Source: CAD feature listing. Evaluate the final solid. Frame: model axes, mm. A direction names the side the tool comes from. Give positions to 0.01 mm unless a question says otherwise; leave off trailing zeros. Loops run counter-clockwise (first coordinate to the right, second up) from the corner with the lowest first, then second, coordinate; pieces in that order, holes last. Notation, with made-up numbers: (-16.5, 16) - (-7.5, 16) arc R33 cw to (-7.5, 48) - close; hole circle Ø7 at (44.25, 74.25). An arc over 180 degrees is marked (long way). Put each result on its own line as item: value.
```python
from build123d import *

# Parameters (mm, degrees)
BASE_FLANGE1_DEPTH              = 3
EDGE_FLANGE1_STRIP_W            = 13.4732
EDGE_FLANGE1_STRIP_H            = 3
EDGE_FLANGE1_STRIP_CUT_DEPTH    = 80
EDGE_FLANGE1_RELIEF_W           = 14.9732
EDGE_FLANGE1_RELIEF_H           = 1.5
EDGE_FLANGE1_RELIEF_CUT_DEPTH   = 3
EDGE_FLANGE1_STRIP_2_W          = 13.4732
EDGE_FLANGE1_STRIP_2_H          = 3
EDGE_FLANGE1_STRIP_CUT_2_DEPTH  = 80
EDGE_FLANGE1_RELIEF_2_W         = 14.9732
EDGE_FLANGE1_RELIEF_2_H         = 1.5
EDGE_FLANGE1_RELIEF_CUT_2_DEPTH = 3
EDGE_FLANGE1_DEPTH              = 80
EDGE_FLANGE1_BEND_DEPTH         = 80
HEM1_START                      = -51.311042424
HEM1_DEPTH                      = 80
HEM1_2_DEPTH                    = 80
EDGE_FLANGE2_STRIP_W            = 13.4732
EDGE_FLANGE2_STRIP_H            = 3
EDGE_FLANGE2_STRIP_CUT_DEPTH    = 80
EDGE_FLANGE2_STRIP_2_W          = 13.4732
EDGE_FLANGE2_STRIP_2_H          = 3
EDGE_FLANGE2_STRIP_CUT_2_DEPTH  = 80
EDGE_FLANGE2_DEPTH              = 80
EDGE_FLANGE2_BEND_DEPTH         = 80
CHAMFER1_SIZE                   = 10
SKETCH24_W                      = 40
SKETCH24_H                      = 20
CUT_EXTRUDE1_DEPTH              = 3
SKETCH25_R                      = 2.58
CUT_EXTRUDE3_DEPTH              = 3
CUT_EXTRUDE2_START              = -3
CUT_EXTRUDE2_OUTLINE_W          = 79.5268
CUT_EXTRUDE2_OUTLINE_H          = 20
CUT_EXTRUDE2_DEPTH              = 3


# Read off the part's stored shape, not the designer's step: Hem1, Cut-Extrude2
# Sheet-metal steps are written as plain solids
with BuildPart() as part:
    # Sketch1 → Base-Flange1 (new body)
    with BuildSketch(Plane(origin=(0, 0, 0), x_dir=(1, 0, 0), z_dir=(0, 1, 0))):
        Polygon((-40.5, 51.311042424), (-40.5, -28.688957576), (40.5, -28.688957576), (40.5, 51.311042424), (40, 51.311042424), (40, 73.311042424), (-40, 73.311042424), (-40, 51.311042424), align=None)
    extrude(amount=-BASE_FLANGE1_DEPTH)

    # Edge-Flange1 strip (across the edge) → Edge-Flange1 strip cut (cut)
    with BuildSketch(Plane(origin=(40.5, 0, 28.688957576), x_dir=(-1, 0, 0), z_dir=(0, 0, -1))):
        with Locations((-6, -1.5)):
            Rectangle(EDGE_FLANGE1_STRIP_W, EDGE_FLANGE1_STRIP_H)
    extrude(amount=EDGE_FLANGE1_STRIP_CUT_DEPTH, mode=Mode.SUBTRACT)

    # Edge-Flange1 relief (on the sheet) → Edge-Flange1 relief cut (cut)
    with BuildSketch(Plane(origin=(39.7634, 0, 28.688957576), x_dir=(-1, 0, 0), z_dir=(0, 1, 0))):
        with Locations((-5.9866, -80.75)):
            Rectangle(EDGE_FLANGE1_RELIEF_W, EDGE_FLANGE1_RELIEF_H)
    extrude(amount=-EDGE_FLANGE1_RELIEF_CUT_DEPTH, mode=Mode.SUBTRACT)

    # Edge-Flange1 strip 2 (across the edge) → Edge-Flange1 strip cut 2 (cut)
    with BuildSketch(Plane(origin=(-40.5, 0, -51.311042424), x_dir=(1, 0, 0), z_dir=(0, 0, 1))):
        with Locations((-6, -1.5)):
            Rectangle(EDGE_FLANGE1_STRIP_2_W, EDGE_FLANGE1_STRIP_2_H)
    extrude(amount=EDGE_FLANGE1_STRIP_CUT_2_DEPTH, mode=Mode.SUBTRACT)

    # Edge-Flange1 relief 2 (on the sheet) → Edge-Flange1 relief cut 2 (cut)
    with BuildSketch(Plane(origin=(-39.7634, 0, -51.311042424), x_dir=(1, 0, 0), z_dir=(0, 1, 0))):
        with Locations((-5.9866, 0.75)):
            Rectangle(EDGE_FLANGE1_RELIEF_2_W, EDGE_FLANGE1_RELIEF_2_H)
    extrude(amount=-EDGE_FLANGE1_RELIEF_CUT_2_DEPTH, mode=Mode.SUBTRACT)

    # Edge-Flange1 section (across the edge) → Edge-Flange1 (add)
    with BuildSketch(Plane(origin=(40.5, 0, 28.688957576), x_dir=(-1, 0, 0), z_dir=(0, 0, -1))):
        with BuildLine():
            Line((-3, 0.7366), (-3, 5))
            Line((-3, 5), (0, 5))
            Line((0, 5), (0, 0.7366))
            ThreePointArc((0, 0.7366), (0.215745145, 0.215745145), (0.7366, 0))
            Line((0.7366, 0), (0.7366, -3))
            ThreePointArc((0.7366, -3), (-1.905575199, -1.905575199), (-3, 0.7366))
        make_face()
    extrude(amount=EDGE_FLANGE1_DEPTH)

    # Edge-Flange1 section 2 (across the edge) → Edge-Flange1 bend (add)
    with BuildSketch(Plane(origin=(-40.5, 0, -51.311042424), x_dir=(1, 0, 0), z_dir=(0, 0, 1))):
        with BuildLine():
            Line((-3, 0.7366), (-3, 5))
            Line((-3, 5), (0, 5))
            Line((0, 5), (0, 0.7366))
            ThreePointArc((0, 0.7366), (0.215745145, 0.215745145), (0.7366, 0))
            Line((0.7366, 0), (0.7366, -3))
            ThreePointArc((0.7366, -3), (-1.905575199, -1.905575199), (-3, 0.7366))
        make_face()
    extrude(amount=EDGE_FLANGE1_BEND_DEPTH)

    # Hem1 outline → Hem1 (cut)
    with BuildSketch(Plane.XY.offset(HEM1_START)):
        with BuildLine():
            ThreePointArc((40.5, 1.95), (41.375718509, 4.088924964), (43.5, 4.999590136))
            Line((43.5, 4.999590136), (43.5, 5))
            Line((43.5, 5), (40.5, 5))
            Line((40.5, 5), (40.5, 1.95))
        make_face()
        with BuildLine():
            Line((-43.5, 5), (-43.5, 4.999590136))
            ThreePointArc((-43.5, 4.999590136), (-41.375718509, 4.088924964), (-40.5, 1.95))
            Line((-40.5, 1.95), (-40.5, 5))
            Line((-40.5, 5), (-43.5, 5))
        make_face()
    extrude(amount=HEM1_DEPTH, mode=Mode.SUBTRACT)

    # Hem1 2 outline → Hem1 2 (add)
    with BuildSketch(Plane.XY.offset(HEM1_START)):
        with BuildLine():
            Line((43.6, -3), (46.6, -3))
            Line((46.6, -3), (46.6, 1.95))
            ThreePointArc((46.6, 1.95), (45.688924964, 4.124281491), (43.5, 4.999590136))
            Line((43.5, 4.999590136), (43.5, 1.95))
            ThreePointArc((43.5, 1.95), (43.55, 2), (43.6, 1.95))
            Line((43.6, 1.95), (43.6, -3))
        make_face()
        with BuildLine():
            Line((-46.6, -3), (-43.6, -3))
            Line((-43.6, -3), (-43.6, 1.95))
            ThreePointArc((-43.6, 1.95), (-43.55, 2), (-43.5, 1.95))
            Line((-43.5, 1.95), (-43.5, 4.999590136))
            ThreePointArc((-43.5, 4.999590136), (-45.688924964, 4.124281491), (-46.6, 1.95))
            Line((-46.6, 1.95), (-46.6, -3))
        make_face()
    extrude(amount=HEM1_2_DEPTH)

    # Edge-Flange2 strip (across the edge) → Edge-Flange2 strip cut (cut)
    with BuildSketch(Plane(origin=(46.6, -3, 28.688957576), x_dir=(0, 1, 0), z_dir=(0, 0, -1))):
        with Locations((-3, -1.5)):
            Rectangle(EDGE_FLANGE2_STRIP_W, EDGE_FLANGE2_STRIP_H)
    extrude(amount=EDGE_FLANGE2_STRIP_CUT_DEPTH, mode=Mode.SUBTRACT)

    # Edge-Flange2 strip 2 (across the edge) → Edge-Flange2 strip cut 2 (cut)
    with BuildSketch(Plane(origin=(-46.6, -3, -51.311042424), x_dir=(0, 1, 0), z_dir=(0, 0, 1))):
        with Locations((-3, -1.5)):
            Rectangle(EDGE_FLANGE2_STRIP_2_W, EDGE_FLANGE2_STRIP_2_H)
    extrude(amount=EDGE_FLANGE2_STRIP_CUT_2_DEPTH, mode=Mode.SUBTRACT)

    # Edge-Flange2 section (across the edge) → Edge-Flange2 (add)
    with BuildSketch(Plane(origin=(46.6, -3, 28.688957576), x_dir=(0, 1, 0), z_dir=(0, 0, -1))):
        with BuildLine():
            Line((0, 0.7366), (0, 56.5))
            Line((0, 56.5), (3, 56.5))
            Line((3, 56.5), (3, 0.7366))
            ThreePointArc((3, 0.7366), (3.215745145, 0.215745145), (3.7366, 0))
            Line((3.7366, 0), (3.7366, -3))
            ThreePointArc((3.7366, -3), (1.094424801, -1.905575199), (0, 0.7366))
        make_face()
    extrude(amount=EDGE_FLANGE2_DEPTH)

    # Edge-Flange2 section 2 (across the edge) → Edge-Flange2 bend (add)
    with BuildSketch(Plane(origin=(-46.6, -3, -51.311042424), x_dir=(0, 1, 0), z_dir=(0, 0, 1))):
        with BuildLine():
            Line((0, 0.7366), (0, 56.5))
            Line((0, 56.5), (3, 56.5))
            Line((3, 56.5), (3, 0.7366))
            ThreePointArc((3, 0.7366), (3.215745145, 0.215745145), (3.7366, 0))
            Line((3.7366, 0), (3.7366, -3))
            ThreePointArc((3.7366, -3), (1.094424801, -1.905575199), (0, 0.7366))
        make_face()
    extrude(amount=EDGE_FLANGE2_BEND_DEPTH)

    # Chamfer1
    chamfer1_edges = [part.edges().sort_by_distance(p)[0] for p in [
        (103.1, -1.5, 28.688957576),
        (103.1, -1.5, -51.311042424),
        (-103.1, -1.5, -51.311042424),
        (-103.1, -1.5, 28.688957576),
    ]]
    chamfer(chamfer1_edges, length=CHAMFER1_SIZE)

    # Sketch24 → Cut-Extrude1 (cut)
    with BuildSketch(Plane(origin=(0, 0, 0), x_dir=(1, 0, 0), z_dir=(0, 1, 0))):
        with Locations((0, 11.311042424)):
            Rectangle(SKETCH24_W, SKETCH24_H)
    extrude(amount=-CUT_EXTRUDE1_DEPTH, mode=Mode.SUBTRACT)

    # Sketch25 → Cut-Extrude3 (cut)
    with BuildSketch(Plane(origin=(0, 0, 0), x_dir=(1, 0, 0), z_dir=(0, 1, 0))):
        with Locations(Location((-30, 61.311042424, 0), (0, 0, 270))):
            Circle(SKETCH25_R)
        with Locations(Location((-10, 61.311042424, 0), (0, 0, 270))):
            Circle(SKETCH25_R)
        with Locations(Location((10, 61.311042424, 0), (0, 0, 270))):
            Circle(SKETCH25_R)
        with Locations(Location((30, 61.311042424, 0), (0, 0, 270))):
            Circle(SKETCH25_R)
        with Locations(Location((30, 41.311042424, 0), (0, 0, 270))):
            Circle(SKETCH25_R)
        with Locations(Location((10, 41.311042424, 0), (0, 0, 270))):
            Circle(SKETCH25_R)
        with Locations(Location((-10, 41.311042424, 0), (0, 0, 270))):
            Circle(SKETCH25_R)
        with Locations(Location((-30, 41.311042424, 0), (0, 0, 270))):
            Circle(SKETCH25_R)
        with Locations(Location((-30, 21.311042424, 0), (0, 0, 270))):
            Circle(SKETCH25_R)
        with Locations(Location((-30, 1.311042424, 0), (0, 0, 270))):
            Circle(SKETCH25_R)
        with Locations(Location((30, 21.311042424, 0), (0, 0, 270))):
            Circle(SKETCH25_R)
        with Locations(Location((30, 1.311042424, 0), (0, 0, 270))):
            Circle(SKETCH25_R)
        with Locations(Location((-93.1, 41.311042424, 0), (0, 0, 270))):
            Circle(SKETCH25_R)
        with Locations(Location((-73.1, 41.311042424, 0), (0, 0, 270))):
            Circle(SKETCH25_R)
        with Locations(Location((-53.1, 41.311042424, 0), (0, 0, 270))):
            Circle(SKETCH25_R)
        with Locations(Location((-93.1, 21.311042424, 0), (0, 0, 270))):
            Circle(SKETCH25_R)
        with Locations(Location((-73.1, 21.311042424, 0), (0, 0, 270))):
            Circle(SKETCH25_R)
        with Locations(Location((-53.1, 21.311042424, 0), (0, 0, 270))):
            Circle(SKETCH25_R)
        with Locations(Location((-93.1, 1.311042424, 0), (0, 0, 270))):
            Circle(SKETCH25_R)
        with Locations(Location((-73.1, 1.311042424, 0), (0, 0, 270))):
            Circle(SKETCH25_R)
        with Locations(Location((-53.1, 1.311042424, 0), (0, 0, 270))):
            Circle(SKETCH25_R)
        with Locations(Location((-53.1, -18.688957576, 0), (0, 0, 270))):
            Circle(SKETCH25_R)
        with Locations(Location((-73.1, -18.688957576, 0), (0, 0, 270))):
            Circle(SKETCH25_R)
        with Locations(Location((-93.1, -18.688957576, 0), (0, 0, 270))):
            Circle(SKETCH25_R)
        with Locations(Location((53.1, 41.311042424, 0), (0, 0, 270))):
            Circle(SKETCH25_R)
        with Locations(Location((73.1, 41.311042424, 0), (0, 0, 270))):
            Circle(SKETCH25_R)
        with Locations(Location((93.1, 41.311042424, 0), (0, 0, 270))):
            Circle(SKETCH25_R)
        with Locations(Location((53.1, 21.311042424, 0), (0, 0, 270))):
            Circle(SKETCH25_R)
        with Locations(Location((73.1, 21.311042424, 0), (0, 0, 270))):
            Circle(SKETCH25_R)
        with Locations(Location((93.1, 21.311042424, 0), (0, 0, 270))):
            Circle(SKETCH25_R)
        with Locations(Location((53.1, 1.311042424, 0), (0, 0, 270))):
            Circle(SKETCH25_R)
        with Locations(Location((73.1, 1.311042424, 0), (0, 0, 270))):
            Circle(SKETCH25_R)
        with Locations(Location((93.1, 1.311042424, 0), (0, 0, 270))):
            Circle(SKETCH25_R)
        with Locations(Location((53.1, -18.688957576, 0), (0, 0, 270))):
            Circle(SKETCH25_R)
        with Locations(Location((73.1, -18.688957576, 0), (0, 0, 270))):
            Circle(SKETCH25_R)
        with Locations(Location((93.1, -18.688957576, 0), (0, 0, 270))):
            Circle(SKETCH25_R)
    extrude(amount=-CUT_EXTRUDE3_DEPTH, mode=Mode.SUBTRACT)

    # Cut-Extrude2 outline → Cut-Extrude2 (cut)
    with BuildSketch(Plane(origin=(0, 0, 0), x_dir=(1, 0, 0), z_dir=(0, 1, 0)).offset(CUT_EXTRUDE2_START)):
        with Locations((0, -18.688957576)):
            Rectangle(CUT_EXTRUDE2_OUTLINE_W, CUT_EXTRUDE2_OUTLINE_H)
    extrude(amount=CUT_EXTRUDE2_DEPTH, mode=Mode.SUBTRACT)


solid = part.part
```
1) Material intervals for line 1 along Z through (x, y) = (4, -1.5); line 2 along Y through (x, z) = (50, -20.5); line 3 along X through (y, z) = (-1.25, -31.5), sorted ascending. Write a range as [from, to].
Check result:
line 1: [-73.31, -21.31], [-1.31, 8.69]
line 2: [-3, 0]
line 3: [-103.1, -44.17], [-42.93, 42.93], [44.17, 103.1]
2) Section query C-C, the plane x = 0. Output: boundary loops of the cut face in (y, z).
Check result:
outline: (-3, -73.31) - (0, -73.31) - (0, -21.31) - (-3, -21.31) - close; (-3, -1.31) - (0, -1.31) - (0, 8.69) - (-3, 8.69) - close
3) Mould query, pull axis X, two halves, no side actions, for faces 3 (the cylindrical face through (-32.29, -1.48, -40.12)), 4 (the flat face through (-75, -3, -12)). Classes: pulls with the +X half, pulls with the -X half, needs draft (parallel to the pull), parting line crosses it, or undercut.
Check result:
face 3: undercut
face 4: needs draft
4) Access query for faces 1 (the cylindrical face through (-72.99, -1.48, 16.11)), 2 (the flat face through (-76, 0, -12)). Directions: +Z, -Z, +X, -X, +Y, -Y. A direction counts if a zero-diameter tool reaches every point of the face in a straight line with its end or side. Return the directions, or none.
Check result:
face 1: +Y, -Y
face 2: +Z, -Z, -X, +Y
5) Section query A-A, the plane x = 53.1. Output: boundary loops of the cut face in (y, z).
Check result:
outline: (-3, -51.31) - (0, -51.31) - (0, -43.89) - (-3, -43.89) - close; (-3, -38.73) - (0, -38.73) - (0, -23.89) - (-3, -23.89) - close; (-3, -18.73) - (0, -18.73) - (0, -3.89) - (-3, -3.89) - close; (-3, 1.27) - (0, 1.27) - (0, 16.11) - (-3, 16.11) - close; (-3, 21.27) - (0, 21.27) - (0, 28.69) - (-3, 28.69) - close
6) Pin query (flat end, axial travel): P1, Ø8, axis at x = -35, z = -56.5, coming from the +Y side; P2, Ø1, axis at y = 2, z = 18.5, coming from the +X side; P3, Ø0.9, axis at x = -11, y = -2, coming from the +Z side. Return the tip coordinate at first contact, or that it passes through.
Check result:
P1: y = 0
P2: x = 46.6
P3: z = 8.69
7) Section query D-D, the plane y = -1.5. State how many separate pieces and enclosed holes the cut face has, plus the area to 3 significant figures.
Check result:
separate pieces: 3
enclosed holes: 37
area: 14,700 mm²
